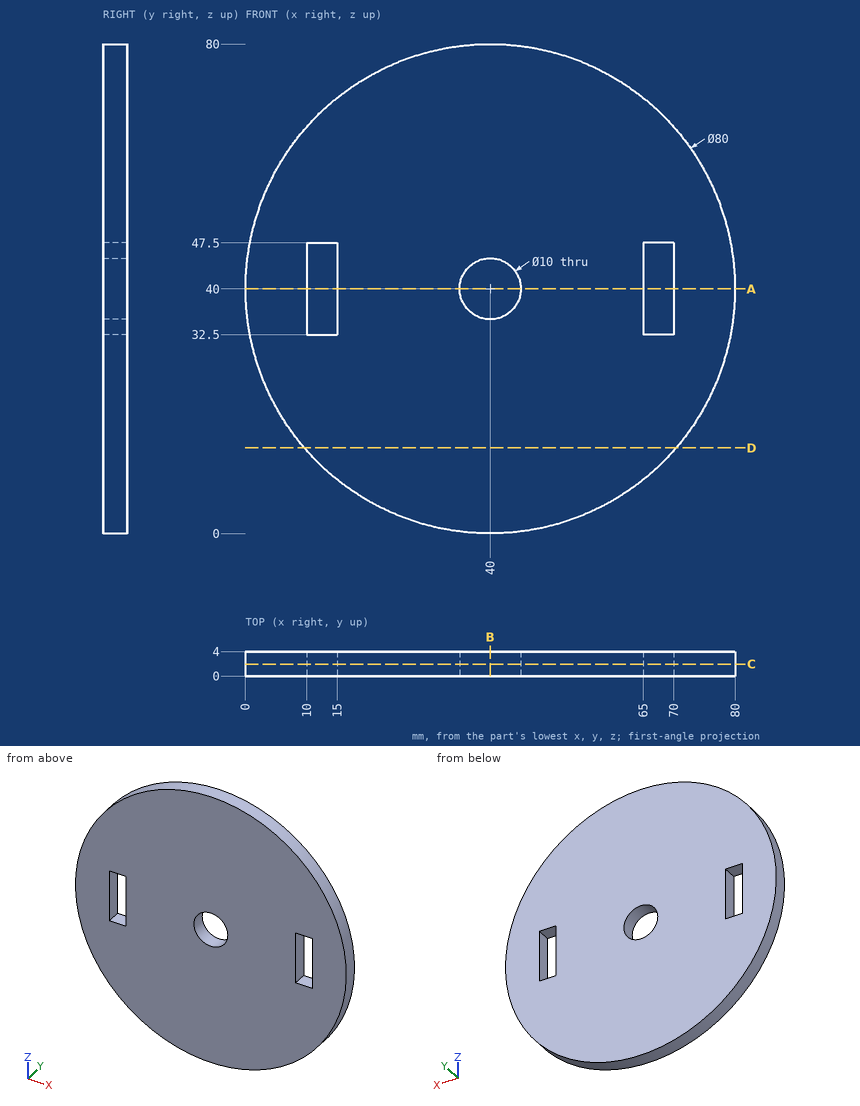
For this review, use the dimensioned drawing (mm, ordinates from the lowest corner) and the shaded views. Round coordinates to 2 decimals unless told otherwise and drop trailing zeros. Order: outer loops, then holes, each group sorted by start corner. A loop starts at its lowest first (then second) coordinate and runs counter-clockwise, first axis right, second up. Notation, with made-up numbers: (43, 70.25) -> (56, 70.25) arc R23 ccw to (56, 82.25) -> close; hole circle Ø1 at (-17.75, 5). An arc over 180 degrees is marked (long way). Write item = value, one per line. Start each with the question number.
Item 1: For line 1 along X through (y, z) = (3, 40); line 2 along X through (y, z) = (1.85, 37); line 3 along Z through (x, y) = (44, 2.3), list the stretches that pass through material, from the lowest coordinate up.
Item 2: Clearance check with flat-ended pins moving along their axes: pin 1 Ø2 at (y, z) = (1.5, 38.5) entering from +X; pin 2 Ø1 at (x, y) = (32.5, 3.5) entering from +Z; pin 3 Ø2 at (y, z) = (0.5, 35.5) entering from +X; pin 4 Ø6 at (x, z) = (40, 40) entering from -Y. State where each tip first meets the part, or that it passes through.
Item 3: Consider section B-B on x = 40. Write out the cut boundary in (y, z), plus the area to 3 significant figures.
Item 4: Consider section A-A on z = 40. Write out the cut boundary in (x, y), plus the area to 3 significant figures.
Item 5: Consider section D-D on z = 14. Write out the cut boundary in (x, y).
Item 6: Consider section C-C on y = 1.95. Write out the cut boundary in (x, z), plus the area to 3 significant figures.
Conclusion:
q1.line_1 = 0 to 10, 15 to 35, 45 to 65, 70 to 80
q1.line_2 = 0.11 to 10, 15 to 36, 44 to 65, 70 to 79.89
q1.line_3 = 0.2 to 37, 43 to 79.8
q2.pin_1 = 80
q2.pin_2 = 79.38
q2.pin_3 = 79.85
q2.pin_4 = through
q3.outline = (0, 0) -> (4, 0) -> (4, 35) -> (0, 35) -> close; (0, 45) -> (4, 45) -> (4, 80) -> (0, 80) -> close
q3.area = 280 mm2
q4.outline = (0, 0) -> (10, 0) -> (10, 4) -> (0, 4) -> close; (15, 0) -> (35, 0) -> (35, 4) -> (15, 4) -> close; (45, 0) -> (65, 0) -> (65, 4) -> (45, 4) -> close; (70, 0) -> (80, 0) -> (80, 4) -> (70, 4) -> close
q4.area = 240 mm2
q5.outline = (9.6, 0) -> (70.4, 0) -> (70.4, 4) -> (9.6, 4) -> close
q6.outline = circle Ø80 at (40, 40); hole (10, 32.5) -> (15, 32.5) -> (15, 47.5) -> (10, 47.5) -> close; hole circle Ø10 at (40, 40); hole (65, 32.5) -> (70, 32.5) -> (70, 47.5) -> (65, 47.5) -> close
q6.area = 4,800 mm2
